```python
from build123d import *

# Parameters (mm, degrees)
F0_W     = 41.91
F0_H     = 5.08
F1_DEPTH = 5.08
F2_DEPTH = 101.6
F3_DEPTH = 63.5
F4_DEPTH = 38.1
F5_R     = 2.53999


# Not quite as in the source:
# - a fillet or chamfer is up to 0.001 mm smaller than in the source, because OpenCascade refuses the exact size


with BuildPart() as f1:
    # F0 (on Top) → F1 (new body)
    with BuildSketch(Plane.XY):
        Polygon((33.655, 9.525), (-33.655, 9.525), (-33.655, 4.445), (-28.575, 4.445), (28.575, 4.445), (33.655, 4.445), align=None)
        Polygon((-28.575, 4.445), (-33.655, 4.445), (-33.655, -9.525), (-20.955, -9.525), (-20.955, -4.445), (-28.575, -4.445), align=None)
        Polygon((33.655, -9.525), (33.655, 4.445), (28.575, 4.445), (28.575, -4.445), (20.955, -4.445), (20.955, -9.525), align=None)
        with Locations((0, -6.985)):
            Rectangle(F0_W, F0_H)
        Polygon((28.575, 4.445), (-28.575, 4.445), (-28.575, -4.445), (-20.955, -4.445), (20.955, -4.445), (28.575, -4.445), align=None)
    extrude(amount=F1_DEPTH)

    # F0 (on Top) → F2 (join)
    with BuildSketch(Plane.XY):
        Polygon((33.655, 9.525), (-33.655, 9.525), (-33.655, 4.445), (-28.575, 4.445), (28.575, 4.445), (33.655, 4.445), align=None)
    extrude(amount=F2_DEPTH)

    # F0 (on Top) → F3 (join)
    with BuildSketch(Plane.XY):
        Polygon((-28.575, 4.445), (-33.655, 4.445), (-33.655, -9.525), (-20.955, -9.525), (-20.955, -4.445), (-28.575, -4.445), align=None)
        Polygon((33.655, -9.525), (33.655, 4.445), (28.575, 4.445), (28.575, -4.445), (20.955, -4.445), (20.955, -9.525), align=None)
    extrude(amount=F3_DEPTH)

    # F0 (on Top) → F4 (join)
    with BuildSketch(Plane.XY):
        with Locations((0, -6.985)):
            Rectangle(F0_W, F0_H)
    extrude(amount=F4_DEPTH)

    # F5 (radius 2.54 in the source; OpenCascade refuses exactly that, so slightly less here)
    f5_edges = [f1.edges().sort_by_distance(p)[0] for p in [
        (-33.655, 4.445, 82.55),
        (33.655, 9.525, 50.8),
        (33.655, 4.445, 82.55),
        (0, 4.445, 101.6),
        (0, 9.525, 101.6),
        (-33.655, 9.525, 50.8),
        (0, 9.525, 0),
        (33.655, -2.54, 63.5),
        (24.765, -4.445, 63.5),
        (28.575, 0, 63.5),
        (27.305, -9.525, 63.5),
        (20.955, -6.985, 63.5),
        (33.655, -9.525, 31.75),
        (20.955, -9.525, 50.8),
        (0, -9.525, 38.1),
        (-20.955, -9.525, 50.8),
        (-20.955, -4.445, 50.8),
        (-27.305, -9.525, 63.5),
        (-24.765, -4.445, 63.5),
        (-28.575, 0, 63.5),
        (-33.655, -2.54, 63.5),
        (-33.655, -9.525, 31.75),
        (0, -9.525, 0),
        (33.655, 0, 0),
        (-33.655, 0, 0),
        (-20.955, -6.985, 63.5),
        (0, -4.445, 38.1),
        (20.955, -4.445, 50.8),
    ]]
    fillet(f5_edges, radius=F5_R)


solid = f1.part
```
Source: CAD feature listing. Evaluate the final solid. Frame: model axes, mm. A direction names the side the tool comes from. Coordinates: 2 decimals unless noted, no trailing zeros. Loops run counter-clockwise (first coordinate to the right, second up) from the corner with the lowest first, then second, coordinate; pieces in that order, holes last. Notation, with made-up numbers: M -4,3.5 L 28,3.5 A25 cw 28,41.5 Z; hole C -23,57.25 d4. An arc over 180 degrees is marked long. Use CSV: the item, a comma, the result in double quotes.
(1) Line query: line 1 (Y direction, x = 5, z = 18) (3 decimals); line 2 (Y direction, x = -3.5, z = 40) (3 decimals); line 3 (X direction, y = 1, z = 20.5) (3 decimals). Output: solid intervals per line, ascending. Write a range as [from, to].
Answers follow:
line 1,"[-9.525, -4.445], [4.445, 9.525]"
line 2,"[4.445, 9.525]"
line 3,"[-33.655, -28.575], [28.575, 33.655]"
(2) Contact query for flat-ended pins moving along their axis: pin 1 (2 mm diameter, centred on x = 8, y = 4, fed in from +Z); pin 2 (3 mm diameter, centred on x = -21.5, z = 68.5, fed in from -Y) (3 decimals); pin 3 (6 mm diameter, centred on x = -25.5, y = 1, fed in from +Z). Output: stop coordinate, or through.
Answers follow:
pin 1,"z = 100.64"
pin 2,"y = 4.445"
pin 3,"z = 5.08"
(3) Reachability of faces 1 (the face through (-32.931, -0.098, 62.736)), 2 (the face through (-21.68, -8.76, 48.44)), 3 (the face through (29.299, -0.08, 62.736)) from +Z, -Z, +X, -X, +Y, -Y: full face, straight path, thin tool, end or side. Return the list, or none.
Answers follow:
face 1,"+Z, -X, -Y"
face 2,"+Z, -Y"
face 3,"+Z"
(4) Cut plane B-B on z = 7.5. Return loops of the section in (x, y) (3 decimals).
Answers follow:
outline,"M -33.655,-6.985 A2.54 ccw -31.115,-9.525 L 31.115,-9.525 A2.54 ccw 33.655,-6.985 L 33.655,6.985 A2.54 ccw 31.115,9.525 L -31.115,9.525 A2.54 ccw -33.655,6.985 Z; hole M -28.575,-4.445 L 28.575,-4.445 L 28.575,4.445 L -28.575,4.445 Z"
(5) Draft query along Y for faces 4 (the face through (-33.655, 0, 29)), 5 (the face through (-0.436, 8.761, 0.724)), 6 (the face through (0, -9.525, 25)), 7 (the face through (0, 0, 5.08)). Return one class per face: pulls with the +Y half, pulls with the -Y half, needs draft (parallel to the pull), parting line crosses it, or undercut.
Answers follow:
face 4,"needs draft"
face 5,"pulls with the +Y half"
face 6,"pulls with the -Y half"
face 7,"undercut"
